Could you check a few things on this drawing? It's one solid part, dimensions in mm from its lowest x, y, z. Round coordinates to 2 decimals unless told otherwise and drop trailing zeros. Write each loop counter-clockwise with the first axis right and the second up, starting at its lowest first coordinate (ties: lowest second). Pieces come first, ordered by that corner, then holes. Notation, with made-up numbers: (20.25, 78) -> (29.25, 78) arc R16 cw to (29.25, 106) -> close; hole circle Ø1 at (82.25, 64). An arc over 180 degrees is marked (long way). Answer in a Markdown table with one row per item.
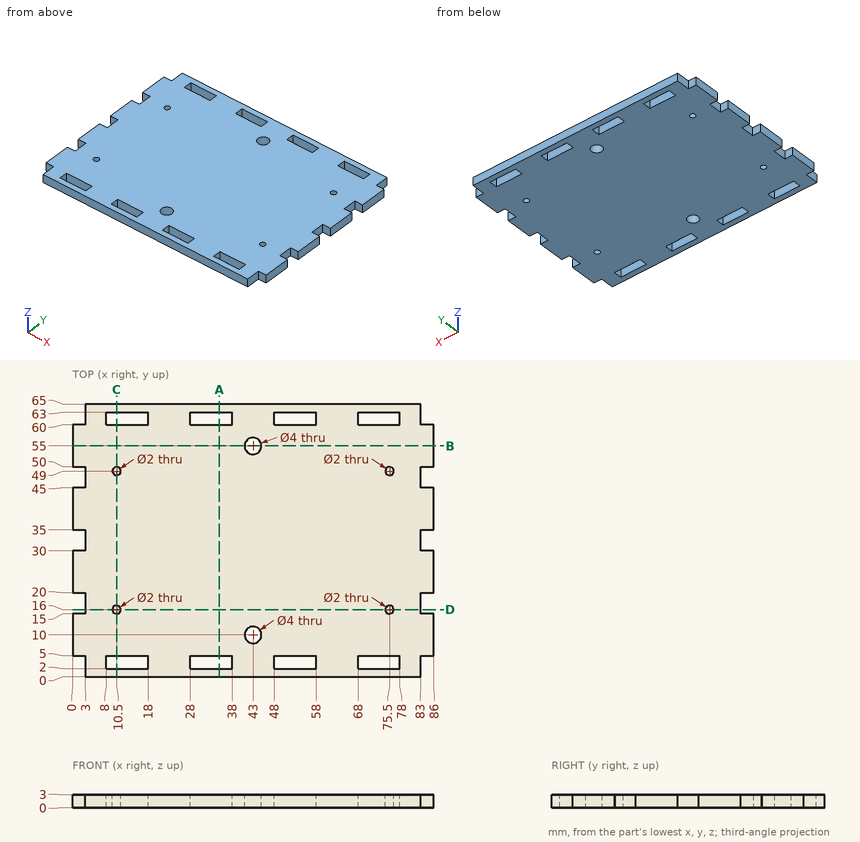
1) For pin 1 (0.9 mm diameter, centred on y = 3, z = 1.5, fed in from -X); pin 2 (0.9 mm diameter, centred on x = 84, z = 1.5, fed in from +Y); pin 3 (0.9 mm diameter, centred on x = 84, z = 1.5, fed in from -Y); pin 4 (3 mm diameter, centred on x = 43, y = 55, fed in from +Z), each with a flat end and sliding along its axis, tell me the tip position at first contact or that it passes through.
Findings:
| item | result |
|---|---|
| pin 1 | stops at x = 3 |
| pin 2 | stops at y = 60 |
| pin 3 | stops at y = 5 |
| pin 4 | passes through |
2) Imagine slicing it at A-A, the plane x = 35. Please give me the cut outline in (y, z), plus the area to 3 significant figures.
Findings:
| item | result |
|---|---|
| outline | (0, 0) -> (2, 0) -> (2, 3) -> (0, 3) -> close; (5, 0) -> (60, 0) -> (60, 3) -> (5, 3) -> close; (63, 0) -> (65, 0) -> (65, 3) -> (63, 3) -> close |
| area | 177 mm^2 |
3) Please list where these lines run through material, in increasing order: line 1 (Y direction, x = 71.5, z = 1.7); line 2 (Y direction, x = 10.5, z = 1.3); line 3 (Y direction, x = 75, z = 1.55).
Findings:
| item | result |
|---|---|
| line 1 | y = 0 to 2, 5 to 60, 63 to 65 |
| line 2 | y = 0 to 2, 5 to 15, 17 to 48, 50 to 60, 63 to 65 |
| line 3 | y = 0 to 2, 5 to 15.13, 16.87 to 48.13, 49.87 to 60, 63 to 65 |
4) Imagine slicing it at D-D, the plane y = 16. Please give me the cut outline in (x, z).
Findings:
| item | result |
|---|---|
| outline | (3, 0) -> (9.5, 0) -> (9.5, 3) -> (3, 3) -> close; (11.5, 0) -> (74.5, 0) -> (74.5, 3) -> (11.5, 3) -> close; (76.5, 0) -> (83, 0) -> (83, 3) -> (76.5, 3) -> close |
5) Imagine slicing it at B-B, the plane y = 55. Please give me the cut outline in (x, z), plus the area to 3 significant figures.
Findings:
| item | result |
|---|---|
| outline | (0, 0) -> (41, 0) -> (41, 3) -> (0, 3) -> close; (45, 0) -> (86, 0) -> (86, 3) -> (45, 3) -> close |
| area | 246 mm^2 |
6) Imagine slicing it at C-C, the plane x = 10.5. Please give me the cut outline in (y, z), plus the area to 3 significant figures.
Findings:
| item | result |
|---|---|
| outline | (0, 0) -> (2, 0) -> (2, 3) -> (0, 3) -> close; (5, 0) -> (15, 0) -> (15, 3) -> (5, 3) -> close; (17, 0) -> (48, 0) -> (48, 3) -> (17, 3) -> close; (50, 0) -> (60, 0) -> (60, 3) -> (50, 3) -> close; (63, 0) -> (65, 0) -> (65, 3) -> (63, 3) -> close |
| area | 165 mm^2 |
